Geometry: final body of the model. Coordinates: model frame, mm. A direction names the side the tool comes from. Coordinates: 2 decimals unless noted, no trailing zeros. Write each loop counter-clockwise with the first axis right and the second up, starting at its lowest first coordinate (ties: lowest second). Pieces come first, ordered by that corner, then holes.
from build123d import *

# Parameters (mm, degrees)
SKETCH1_R           = 13.5
BOSS_EXTRUDE1_DEPTH = 19
BOSS_EXTRUDE2_START = 19
SKETCH1_3_R         = 11.125
BOSS_EXTRUDE2_DEPTH = 7.6
BOSS_EXTRUDE3_START = 26.6
SKETCH1_4_R         = 9.75
BOSS_EXTRUDE3_DEPTH = 17.1
BOSS_EXTRUDE4_START = 19
SKETCH1_5_R         = 2.08
BOSS_EXTRUDE4_DEPTH = 6
CHAMFER1_SIZE       = 1


with BuildPart() as part:
    # Sketch1 → Boss-Extrude1 (new body)
    with BuildSketch(Plane(origin=(0, 0, 0), x_dir=(1, 0, 0), z_dir=(0, 1, 0))):
        Circle(SKETCH1_R)
    extrude(amount=BOSS_EXTRUDE1_DEPTH)

    # Sketch1<3> → Boss-Extrude2 (add)
    with BuildSketch(Plane(origin=(0, 0, 0), x_dir=(1, 0, 0), z_dir=(0, 1, 0)).offset(BOSS_EXTRUDE2_START)):
        Circle(SKETCH1_3_R)
    extrude(amount=BOSS_EXTRUDE2_DEPTH)

    # Sketch1<4> → Boss-Extrude3 (add)
    with BuildSketch(Plane(origin=(0, 0, 0), x_dir=(1, 0, 0), z_dir=(0, 1, 0)).offset(BOSS_EXTRUDE3_START)):
        Circle(SKETCH1_4_R)
    extrude(amount=BOSS_EXTRUDE3_DEPTH)

    # Sketch1<5> → Boss-Extrude4 (add)
    with BuildSketch(Plane(origin=(0, 0, 0), x_dir=(1, 0, 0), z_dir=(0, 1, 0)).offset(BOSS_EXTRUDE4_START)):
        with BuildLine():
            ThreePointArc((5.25, 18.912204045), (0, 23.2511033), (-5.25, 18.912204045))
            Line((-5.25, 18.912204045), (-6.620548595, 11.765132227))
            ThreePointArc((-6.620548595, 11.765132227), (0, 13.5), (6.620548595, 11.765132227))
            Line((6.620548595, 11.765132227), (5.25, 18.912204045))
        make_face()
        with Locations((0, 18.912204045)):
            Circle(SKETCH1_5_R, mode=Mode.SUBTRACT)
    extrude(amount=-BOSS_EXTRUDE4_DEPTH)

    # Chamfer1
    chamfer1_edges = [part.edges().sort_by_distance(p)[0] for p in [
        (0, 13, -23.2511033),
        (5.935274297, 13, -15.338668136),
        (-5.935274297, 13, -15.338668136),
    ]]
    chamfer(chamfer1_edges, length=CHAMFER1_SIZE)


solid = part.part
Item 1: Section B-B, the plane z = 0. Output: boundary loops of the cut face in (x, y) (3 decimals).
Derived:
outline: (-13.5, 0) - (13.5, 0) - (13.5, 19) - (11.125, 19) - (11.125, 26.6) - (9.75, 26.6) - (9.75, 43.7) - (-9.75, 43.7) - (-9.75, 26.6) - (-11.125, 26.6) - (-11.125, 19) - (-13.5, 19) - close
Item 2: Pull-direction query (X, two-part tool) for faces 3 (the flat face through (0, 0, 0)), 4 (the cylindrical face through (-0.45, 16.04, -16.88)), 5 (the flat face through (5.461, 13.507, -15.196)); classes: released by +X, released by -X, zero draft, split by the parting line, or undercut.
Derived:
face 3: zero draft
face 4: undercut
face 5: released by +X
Item 3: Set-up query: faces 1 (the cylindrical face through (-8.2, 22.75, -7.52)), 2 (the flat face through (0, 43.7, 0)). Return all of +Z, -Z, +X, -X, +Y, -Y with unobstructed straight access to the full face (end or side cutting, diameter ignored); none if empty.
Derived:
face 1: +Y
face 2: +Z, -Z, +X, -X, +Y
Item 4: Pin query (flat end, axial travel): pin 1 (6 mm diameter, centred on y = 13, z = -14.5, fed in from -X); pin 2 (1 mm diameter, centred on x = 3.5, y = 12.5, fed in from +Z); pin 3 (5 mm diameter, centred on x = 0, z = -18.91, fed in from -Y). Return the tip coordinate at first contact, or that it passes through.
Derived:
pin 1: stops at x = -7.07
pin 2: stops at z = 13.16
pin 3: stops at y = 13
Item 5: Section A-A, the plane x = 0. Output: boundary loops of the cut face in (y, z) (3 decimals), plus the area to 3 significant figures.
Derived:
outline: (0, -13.5) - (13, -13.5) - (13, -16.832) - (19, -16.832) - (19, -11.125) - (26.6, -11.125) - (26.6, -9.75) - (43.7, -9.75) - (43.7, 9.75) - (26.6, 9.75) - (26.6, 11.125) - (19, 11.125) - (19, 13.5) - (0, 13.5) - close; (13, -22.251) - (14, -23.251) - (19, -23.251) - (19, -20.992) - (13, -20.992) - close
area: 1,050 mm2
Item 6: Section D-D, the plane x = 8.75. Output: boundary loops of the cut face in (y, z), plus the area to 3 significant figures.
Derived:
outline: (0, -10.28) - (19, -10.28) - (19, -6.87) - (26.6, -6.87) - (26.6, -4.3) - (43.7, -4.3) - (43.7, 4.3) - (26.6, 4.3) - (26.6, 6.87) - (19, 6.87) - (19, 10.28) - (0, 10.28) - close
area: 642 mm2
Item 7: Section C-C, the plane y = 4. Output: boundary loops of the cut face in (x, z).
Derived:
outline: circle Ø27 at (0, 0)
Item 8: Material intervals for probe 1 along Z at (x, y) = (0, 17.7); probe 2 along Y at (x, z) = (-2, -10.5); probe 3 along Z at (x, y) = (0.25, 19.5), sorted ascending.
Derived:
probe 1: z = -23.25 to -20.99, -16.83 to 13.5
probe 2: y = 0 to 26.6
probe 3: z = -11.12 to 11.12
